from build123d import *

# Parameters (mm, degrees)
SKETCH18_R          = 3.175
SKETCH18_R_2        = 6.35
SKETCH18_R_3        = 2.5019
BOSS_EXTRUDE4_DEPTH = 6.35
CHAMFER1_SIZE       = 2.54
SKETCH19_R          = 4
CUT_EXTRUDE1_DEPTH  = 43.434


with BuildPart() as part:
    # Sketch18 → Boss-Extrude4 (new body)
    with BuildSketch(Plane.XY):
        with BuildLine():
            Line((0, 0), (-265.604745697, 0))
            ThreePointArc((-265.604745697, 0), (-298.882523776, 76.131915965), (-307.699061234, 158.75))
            Line((-307.699061234, 158.75), (-307.699061234, 165.1))
            ThreePointArc((-307.699061234, 165.1), (-305.839189294, 169.590128061), (-301.349061234, 171.45))
            Line((-301.349061234, 171.45), (-231.499061234, 171.45))
            Line((-231.499061234, 171.45), (-159.473782125, 158.75))
            Line((-159.473782125, 158.75), (-28.014368889, 158.75))
            ThreePointArc((-28.014368889, 158.75), (-23.851207857, 157.194850386), (-21.727208485, 153.291130779))
            Line((-21.727208485, 153.291130779), (0, 0))
        make_face()
        with Locations((-11.423473622, 24.034728138)):
            Circle(SKETCH18_R, mode=Mode.SUBTRACT)
        with Locations((-27.253356194, 124.406511892)):
            Circle(SKETCH18_R, mode=Mode.SUBTRACT)
        with Locations((-35.200938766, 146.05)):
            Circle(SKETCH18_R_2, mode=Mode.SUBTRACT)
        with Locations((-301.900938766, 146.05)):
            Circle(SKETCH18_R, mode=Mode.SUBTRACT)
        with Locations((-301.569673588, 132.761391752)):
            Circle(SKETCH18_R, mode=Mode.SUBTRACT)
        with Locations((-300.579872803, 119.537524267)):
            Circle(SKETCH18_R, mode=Mode.SUBTRACT)
        with Locations((-298.943543444, 106.442822899)):
            Circle(SKETCH18_R, mode=Mode.SUBTRACT)
        with Locations((-239.568937637, 24.034728138)):
            Circle(SKETCH18_R, mode=Mode.SUBTRACT)
        with Locations((-286.962142025, 164.850708953)):
            Circle(SKETCH18_R, mode=Mode.SUBTRACT)
        with Locations((-165.1, 146.05)):
            Circle(SKETCH18_R_3, mode=Mode.SUBTRACT)
        with Locations((-143.102954744, 107.95)):
            Circle(SKETCH18_R_3, mode=Mode.SUBTRACT)
        with Locations((-187.097045256, 107.95)):
            Circle(SKETCH18_R_3, mode=Mode.SUBTRACT)
    extrude(amount=BOSS_EXTRUDE4_DEPTH)

    # Chamfer1
    chamfer1_edges = [part.edges().sort_by_distance(p)[0] for p in [
        (-14.598473622, 24.034728138, 6.35),
        (-30.428356194, 124.406511892, 6.35),
        (-242.743937637, 24.034728138, 6.35),
        (-290.137142025, 164.850708953, 6.35),
    ]]
    chamfer(chamfer1_edges, length=CHAMFER1_SIZE)

    # Sketch19 → Cut-Extrude1 (cut)
    with BuildSketch(Plane(origin=(0, 0, 0), x_dir=(-1, 0, 0), z_dir=(0, 0, -1))):
        with Locations((86.747156029, 87.953133026)):
            Circle(SKETCH19_R)
    extrude(amount=-CUT_EXTRUDE1_DEPTH, mode=Mode.SUBTRACT)


solid = part.part
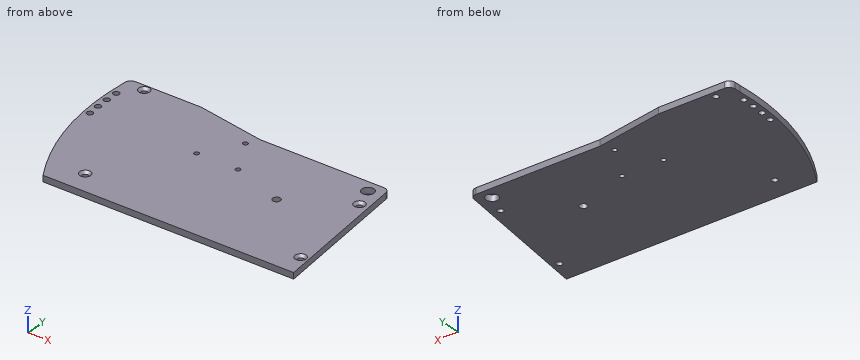
Geometry check sheet. Reference: the model listing, model coordinates, mm. Give positions to 0.01 mm unless a question says otherwise; leave off trailing zeros. Write each loop counter-clockwise with the first axis right and the second up, starting at its lowest first coordinate (ties: lowest second). Pieces come first, ordered by that corner, then holes.
1) Go/stop test with flat-tipped pins: pin 1 Ø4 at (x, y) = (-27.25, 124.41) entering from +Z; pin 2 Ø1.5 at (y, z) = (114, 2) entering from -X; pin 3 Ø7.5 at (x, y) = (-239.57, 24.03) entering from +Z; pin 4 Ø1.9 at (y, z) = (163, 3) entering from -X. Record where each tip stops, or that it passes through.
Values follow:
pin 1: passes through
pin 2: stops at x = -306.19
pin 3: stops at z = 4.39
pin 4: stops at x = -307.7
2) Cross-section at B-B (y = 53.5). Record the boundary of the cut face in (x, z), plus the area to 3 significant figures.
Values follow:
outline: (-291.82, 0) - (-7.58, 0) - (-7.58, 6.35) - (-291.82, 6.35) - close
area: 1,800 mm2
3) Thickness scan on line 1 (X direction, y = 20, z = 6); line 2 (X direction, y = 148, z = 2.25); line 3 (Y direction, x = -188, z = 3.5). Record the ranges inside material, lowest first.
Values follow:
line 1: x = -277.13 to -243.11, -236.03 to -14.96, -7.89 to -2.83
line 2: x = -307.99 to -304.41, -299.4 to -166.67, -163.53 to -41.24, -29.16 to -20.98
line 3: y = 0 to 105.62, 110.28 to 163.78
4) Cross-section at A-A (x = -55). Record the boundary of the cut face in (y, z), plus the area to 3 significant figures.
Values follow:
outline: (0, 0) - (158.75, 0) - (158.75, 6.35) - (0, 6.35) - close
area: 1,010 mm2
